Source: CAD feature listing. Evaluate the final solid. Frame: model axes, mm. A direction names the side the tool comes from. Give positions to 0.01 mm unless a question says otherwise; leave off trailing zeros. Loops run counter-clockwise (first coordinate to the right, second up) from the corner with the lowest first, then second, coordinate; pieces in that order, holes last. Notation, with made-up numbers: (18.5, 34) -> (32.5, 34) arc R13 cw to (32.5, 47) -> close; hole circle Ø2 at (15.25, 5). An arc over 180 degrees is marked (long way). Put each result on its own line as item: value.
```python
from build123d import *

# Parameters (mm, degrees)
F0_R     = 9.525
F1_DEPTH = 25.4
F3_DEPTH = 25.401
F4_DEPTH = 11.0998
F6_DEPTH = 9.525


with BuildPart() as f1:
    # F0 (on Top) → F1 (new body)
    with BuildSketch(Plane.XY):
        Circle(F0_R)
    extrude(amount=F1_DEPTH)

    # F2 (on Top) → F3 (cut, through all)
    with BuildSketch(Plane.XY):
        with BuildLine():
            ThreePointArc((-4.7625, 0), (-3.367596, -3.367596), (0, -4.7625))
            ThreePointArc((0, -4.7625), (3.367596, -3.367596), (4.7625, 0))
            ThreePointArc((4.7625, 0), (3.367596, 3.367596), (0, 4.7625))
            ThreePointArc((0, 4.7625), (-3.367596, 3.367596), (-4.7625, 0))
        make_face()
    extrude(amount=F3_DEPTH, mode=Mode.SUBTRACT)

    # F2 (on Top) → F4 (cut)
    with BuildSketch(Plane.XY):
        with BuildLine():
            Line((0, -4.7625), (4.7625, -4.7625))
            Line((4.7625, -4.7625), (4.7625, 0))
            ThreePointArc((4.7625, 0), (3.367596, -3.367596), (0, -4.7625))
        make_face()
        with BuildLine():
            Line((-4.7625, -4.7625), (0, -4.7625))
            ThreePointArc((0, -4.7625), (-3.367596, -3.367596), (-4.7625, 0))
            Line((-4.7625, 0), (-4.7625, -4.7625))
        make_face()
        with BuildLine():
            ThreePointArc((0, 4.7625), (3.367596, 3.367596), (4.7625, 0))
            Line((4.7625, 0), (4.7625, 4.7625))
            Line((4.7625, 4.7625), (0, 4.7625))
        make_face()
        with BuildLine():
            Line((-4.7625, 4.7625), (-4.7625, 0))
            ThreePointArc((-4.7625, 0), (-3.367596, 3.367596), (0, 4.7625))
            Line((0, 4.7625), (-4.7625, 4.7625))
        make_face()
    extrude(amount=F4_DEPTH, mode=Mode.SUBTRACT)

    # F5 (on face) → F6 (cut)
    with BuildSketch(Plane.XY.offset(25.4)):
        Polygon((0.103503, -7.3025), (6.375902, -3.561614), (6.272399, 3.740886), (-0.103503, 7.3025), (-6.375902, 3.561614), (-6.272399, -3.740886), align=None)
    extrude(amount=-F6_DEPTH, mode=Mode.SUBTRACT)


solid = f1.part
```
(1) Section C-C on x = 3.5. Return loops of the section in (y, z) (1 decimal), then the cut area to 3 significant figures.
Calculated:
outline: (-8.9, 0) -> (-4.8, 0) -> (-4.8, 11.1) -> (-3.2, 11.1) -> (-3.2, 15.9) -> (-5.3, 15.9) -> (-5.3, 25.4) -> (-8.9, 25.4) -> close; (3.2, 11.1) -> (4.8, 11.1) -> (4.8, 0) -> (8.9, 0) -> (8.9, 25.4) -> (5.3, 25.4) -> (5.3, 15.9) -> (3.2, 15.9) -> close
area: 213 mm²
(2) Draft query along Y for faces 1 (the flat face through (-2.3, -6.2, 25.4)), 2 (the cylindrical face through (-7.559, -5.796, 12.522)), 3 (the flat face through (4, -4, 11.1)). Return one class per face: released by +Y, released by -Y, zero draft, split by the parting line, or undercut.
Calculated:
face 1: zero draft
face 2: split by the parting line
face 3: undercut
(3) Reachability of faces 4 (the flat face through (0, -6, 0)), 5 (the flat face through (-3.196, 5.458, 20.704)), 6 (the flat face through (0, -4.762, 5)) from +Z, -Z, +X, -X, +Y, -Y: full face, straight path, thin tool, end or side. Return the list, or none.
Calculated:
face 4: -Z, +X, -X, +Y, -Y
face 5: +Z
face 6: -Z
(4) Line query: probe 1 along Z at (x, y) = (5.25, -2.5) (3 decimals); probe 2 along Y at (x, z) = (-0.5, 21.25); probe 3 along Y at (x, z) = (-3.25, 18.25). Output: solid intervals per line, ascending. Write a range as from..to.
Calculated:
probe 1: z = 0..15.875
probe 2: y = -9.51..-6.97, 7.07..9.51
probe 3: y = -8.95..-5.43, 5.43..8.95
(5) First-contact query: P1, Ø2.5, axis at x = -3, y = 2.5, coming from the -Z side; P2, Ø3, axis at x = 1, y = 4, coming from the +Z side (3 decimals); P3, Ø3, axis at y = 4, z = 5, coming from the -X side; P4, Ø1.4, axis at x = 2, y = -3, coming from the -Z side. Flat tips, straight axial feed; report the tip coordinate or a pass-through.
Calculated:
P1: stops at z = 11.1
P2: stops at z = 15.875
P3: stops at x = -9.19
P4: passes through
